from build123d import *

# Parameters (mm, degrees)
SKETCH_1_W                 = 112.5
SKETCH_1_H                 = 13
EXTRUDE_1_DEPTH            = 4
EXTRUDE_2_DEPTH            = 4
SKETCH_3_W                 = 109.5
SKETCH_3_H                 = 10
CUT_EXTRUDE_1_DEPTH        = 2
CUT_EXTRUDE_2_REACH        = 61.142
PATTERN_LINEAR_1_COUNT     = 4
PATTERN_LINEAR_1_PITCH     = 15
PATTERN_LINEAR_1_COL_COUNT = 3
PATTERN_LINEAR_1_COL_PITCH = 15
FILLET_1_R                 = 0.1


with BuildPart() as part:
    # 草图1 → 凸台-拉伸1 (new body)
    with BuildSketch(Plane(origin=(0, 0, 0), x_dir=(1, 0, 0), z_dir=(0, 1, 0))):
        Rectangle(SKETCH_1_W, SKETCH_1_H)
    extrude(amount=EXTRUDE_1_DEPTH)

    # 草图2 → 凸台-拉伸2 (add)
    with BuildSketch(Plane.XZ):
        with BuildLine():
            Line((56.25, -1.5), (56.25, 1.5))
            Line((56.25, 1.5), (56.927124344, 1.5))
            ThreePointArc((56.927124344, 1.5), (57.338161527, 1.780042303), (57.805590279, 1.95))
            Line((57.805590279, 1.95), (58.75, 1.95))
            Line((58.75, 1.95), (58.75, -1.95))
            Line((58.75, -1.95), (57.805590279, -1.95))
            ThreePointArc((57.805590279, -1.95), (57.338161527, -1.780042303), (56.927124344, -1.5))
            Line((56.927124344, -1.5), (56.25, -1.5))
        make_face()
    extrude_2 = extrude(amount=-EXTRUDE_2_DEPTH)

    # 镜向1: 凸台-拉伸2 across plane
    add(extrude_2.mirror(Plane(origin=(0, 0, 0), x_dir=(0, 0, 1), z_dir=(1, 0, 0))))

    # 草图3 → 切除-拉伸1 (cut)
    with BuildSketch(Plane(origin=(0, 4, 0), x_dir=(1, 0, 0), z_dir=(0, 1, 0))):
        Rectangle(SKETCH_3_W, SKETCH_3_H)
    extrude(amount=-CUT_EXTRUDE_1_DEPTH, mode=Mode.SUBTRACT)

    # 草图4 → 切除-拉伸2 (cut, up to next)
    with BuildSketch(Plane(origin=(0, 2, 0), x_dir=(1, 0, 0), z_dir=(0, 1, 0)), mode=Mode.PRIVATE) as cut_extrude_2_sk1:
        with BuildLine():
            Line((-4, -2.5), (-4, 0.5))
            Line((-4, 0.5), (-6.177124344, 0.5))
            ThreePointArc((-6.177124344, 0.5), (-7.5, 1), (-8.822875656, 0.5))
            Line((-8.822875656, 0.5), (-11, 0.5))
            Line((-11, 0.5), (-11, -2.5))
            Line((-11, -2.5), (-8.822875656, -2.5))
            ThreePointArc((-8.822875656, -2.5), (-7.5, -3), (-6.177124344, -2.5))
            Line((-6.177124344, -2.5), (-4, -2.5))
        make_face()
    cut_extrude_2_tool1 = extrude(cut_extrude_2_sk1.sketch, amount=-CUT_EXTRUDE_2_REACH, mode=Mode.PRIVATE) & part.part
    cut_extrude_2 = cut_extrude_2_tool1.solids().sort_by_distance((-7.5, 2, 1))[0]
    add(cut_extrude_2, mode=Mode.SUBTRACT)

    # 阵列(线性)1: 切除-拉伸2 ×4
    with Locations(*[(i * PATTERN_LINEAR_1_PITCH, 0, 0) for i in range(1, PATTERN_LINEAR_1_COUNT)]):
        add(cut_extrude_2, mode=Mode.SUBTRACT)

    # 阵列(线性)1 col: 切除-拉伸2 ×3
    with Locations(*[(-i * PATTERN_LINEAR_1_COL_PITCH, 0, 0) for i in range(1, PATTERN_LINEAR_1_COL_COUNT)]):
        add(cut_extrude_2, mode=Mode.SUBTRACT)

    # 圆角1
    fillet_1_edges = [part.edges().sort_by_distance(p)[0] for p in [
        (58.75, 2, -1.95),
        (58.75, 2, 1.95),
        (-58.75, 2, -1.95),
        (-58.75, 2, 1.95),
    ]]
    fillet(fillet_1_edges, radius=FILLET_1_R)


solid = part.part
Check sheet for the modelled part. Datum: model origin and axes. Units: mm. A direction names the side the tool comes from. Round coordinates to 2 decimals unless told otherwise and drop trailing zeros. Write each loop counter-clockwise with the first axis right and the second up, starting at its lowest first coordinate (ties: lowest second). Pieces come first, ordered by that corner, then holes. Notation, with made-up numbers: (87.5, -5.5) -> (92.5, -5.5) arc R12 cw to (92.5, 9.5) -> close; hole circle Ø4 at (5, 19.25). An arc over 180 degrees is marked (long way). Answer as CSV lines item,"result". Start each with the question number.
1) Section check B-B on y = 3.4. Enter the section's corners in (x, z).
2) Tool access check on faces 1 (the cylindrical face through (-22.5, 1, -1)), 2 (the flat face through (-1, 2, 0)). Record the directions out of +Z, -Z, +X, -X, +Y, -Y that give a thin tool (end or side, any length) a straight path to the whole face; none if there is none.
3) Section check C-C on z = -3. Enter the section's corners in (x, y), and give its area (3 significant figures).
4) Section check A-A on x = 5. Enter the section's corners in (y, z), and give its area (3 significant figures).
5) Go/stop test with flat-tipped pins: P1, Ø5, axis at x = -13, z = -4, coming from the +Y side; P2, Ø1.2, axis at y = 2, z = -5, coming from the -X side; P3, Ø3, axis at x = 17.5, z = 1, coming from the +Y side. Record where each tip stops, or that it passes through.
6) Material ranges on line 1 (Z direction, x = 18, y = 2.15); line 2 (X direction, y = 3.8, z = 1); line 3 (Y direction, x = -1, z = 2.75), recorded low to high. Write a range as from..to.
7) Release check for a two-part mould opening along Z. For faces 3 (the flat face through (-1, 2, -6.5)), 4 (the flat face through (-25, 1, 2.5)), 5 (the flat face through (58.75, 2, 0)) record: pulls with the +Z half, pulls with the -Z half, needs draft (parallel to the pull), parting line crosses it, or undercut.
Found:
1,outline,"(-58.75, -1.85) arc R0.1 ccw to (-58.65, -1.95) -> (-57.81, -1.95) arc R2 ccw to (-56.93, -1.5) -> (-56.25, -1.5) -> (-56.25, -6.5) -> (56.25, -6.5) -> (56.25, -1.5) -> (56.93, -1.5) arc R2 ccw to (57.81, -1.95) -> (58.65, -1.95) arc R0.1 ccw to (58.75, -1.85) -> (58.75, 1.85) arc R0.1 ccw to (58.65, 1.95) -> (57.81, 1.95) arc R2 ccw to (56.93, 1.5) -> (56.25, 1.5) -> (56.25, 6.5) -> (-56.25, 6.5) -> (-56.25, 1.5) -> (-56.93, 1.5) arc R2 ccw to (-57.81, 1.95) -> (-58.65, 1.95) arc R0.1 ccw to (-58.75, 1.85) -> close; hole (-54.75, -5) -> (54.75, -5) -> (54.75, 5) -> (-54.75, 5) -> close"
2,face 1,"+Y, -Y"
2,face 2,"+Y"
3,outline,"(-56.25, 0) -> (56.25, 0) -> (56.25, 4) -> (54.75, 4) -> (54.75, 2) -> (-54.75, 2) -> (-54.75, 4) -> (-56.25, 4) -> close"
3,area,"231 mm^2"
4,outline,"(0, -6.5) -> (4, -6.5) -> (4, -5) -> (2, -5) -> (2, -0.5) -> (0, -0.5) -> close; (0, 2.5) -> (2, 2.5) -> (2, 5) -> (4, 5) -> (4, 6.5) -> (0, 6.5) -> close"
4,area,"26.0 mm^2"
5,P1,"stops at y = 4"
5,P2,"stops at x = -56.25"
5,P3,"stops at y = 2"
6,line 1,"z = -6.5..-5, 5..6.5"
6,line 2,"x = -58.75..-54.75, 54.75..58.75"
6,line 3,"y = 0..2"
7,face 3,"pulls with the -Z half"
7,face 4,"undercut"
7,face 5,"needs draft"
